Source: CAD feature listing. Evaluate the final solid. Frame: model axes, mm. A direction names the side the tool comes from. Give positions to 0.01 mm unless a question says otherwise; leave off trailing zeros. Loops run counter-clockwise (first coordinate to the right, second up) from the corner with the lowest first, then second, coordinate; pieces in that order, holes last. Notation, with made-up numbers: M 85,46 L 137,46 A15 cw 137,73 Z; hole C -26,73.5 d2. An arc over 180 degrees is marked long. Answer in a Markdown table with one row per item.
```python
from build123d import *

# Parameters (mm, degrees)
F0_R     = 6.35
F1_DEPTH = 12.7
F2_W     = 3.81
F2_H     = 3.81
F3_DEPTH = 25.4


with BuildPart() as f1:
    # F0 (on Front) → F1 (new body, symmetric)
    with BuildSketch(Plane.XZ):
        Circle(F0_R)
    extrude(amount=F1_DEPTH, both=True)

    # F2 (on Top) → F3 (join)
    with BuildSketch(Plane.XY):
        with Locations((0, 7.143756)):
            Rectangle(F2_W, F2_H)
    extrude(amount=F3_DEPTH)


solid = f1.part
```
1) Set-up query: faces 1 (the flat face through (0, 12.7, 0)), 2 (the flat face through (-1.905, 7, 16)), 3 (the flat face through (1.905, 7, 16)). Return all of +Z, -Z, +X, -X, +Y, -Y with unobstructed straight access to the full face (end or side cutting, diameter ignored); none if empty.
Reply:
| item | result |
|---|---|
| face 1 | +Z, -Z, +X, -X, +Y |
| face 2 | +Z, -X, +Y, -Y |
| face 3 | +Z, +X, +Y, -Y |
2) Section B-B, the plane y = 0.25. Return loops of the section in (x, z), then the cut area to 3 significant figures.
Reply:
| item | result |
|---|---|
| outline | C 0,0 d12.7 |
| area | 127 mm² |
3) Pin query (flat end, axial travel): pin 1 Ø4 at (y, z) = (1.5, -1) entering from -X; pin 2 Ø1.5 at (y, z) = (7, 7.5) entering from +X (3 decimals); pin 3 Ø6 at (x, y) = (4.5, -2) entering from +Z; pin 4 Ø4 at (y, z) = (7, 20.5) entering from -X (3 decimals). Return the tip coordinate at first contact, or that it passes through.
Reply:
| item | result |
|---|---|
| pin 1 | stops at x = -6.35 |
| pin 2 | stops at x = 1.905 |
| pin 3 | stops at z = 6.17 |
| pin 4 | stops at x = -1.905 |
4) Section A-A, the plane x = 0. Return loops of the section in (y, z), then the cut area to 3 significant figures.
Reply:
| item | result |
|---|---|
| outline | M -12.7,-6.35 L 12.7,-6.35 L 12.7,6.35 L 9.05,6.35 L 9.05,25.4 L 5.24,25.4 L 5.24,6.35 L -12.7,6.35 Z |
| area | 395 mm² |
5) Material intervals for L1, parallel to Z at x = -0.25, y = -10; L2, parallel to Z at x = 2.75, y = 4; L3, parallel to Y at x = 1.5, z = 16, sorted ascending.
Reply:
| item | result |
|---|---|
| L1 | z = -6.35 to 6.35 |
| L2 | z = -5.72 to 5.72 |
| L3 | y = 5.24 to 9.05 |
6) Section C-C, the plane z = 12. Return loops of the section in (x, y) (3 decimals).
Reply:
| item | result |
|---|---|
| outline | M -1.905,5.239 L 1.905,5.239 L 1.905,9.049 L -1.905,9.049 Z |
7) Section D-D, the plane z = -1.5. Return loops of the section in (x, y).
Reply:
| item | result |
|---|---|
| outline | M -6.17,-12.7 L 6.17,-12.7 L 6.17,12.7 L -6.17,12.7 Z |
